Could you check a few things on this model? Use its own coordinates, in mm. Face numbers are marked on the shaded views. Round coordinates to 2 decimals unless told otherwise and drop trailing zeros. Order: outer loops, then holes, each group sorted by start corner. A loop starts at its lowest first (then second) coordinate and runs counter-clockwise, first axis right, second up. Notation, with made-up numbers: (-17, 54.25) - (-11, 54.25) arc R20 ccw to (-11, 79.25) - close; hole circle Ø1 at (21.25, -40). An arc over 180 degrees is marked (long way). Return JSON: item names as keys, results as strings. Group by question number.
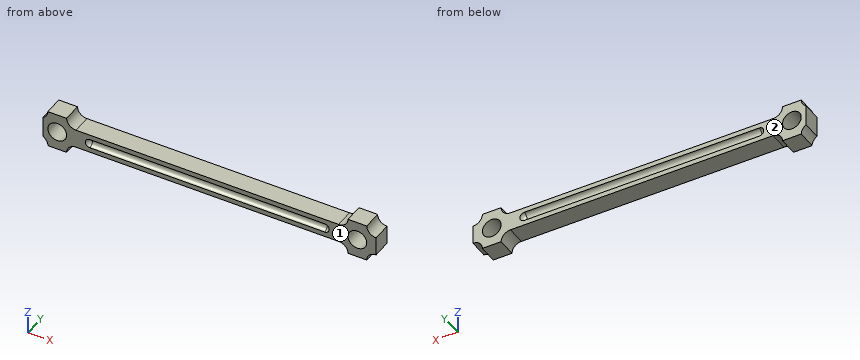
from build123d import *

# Parameters (mm, degrees)
F0_R     = 3.175
F1_DEPTH = 3.175
F3_DEPTH = 41.275
F4_R     = 1.52399


# Not quite as in the source:
# - a fillet or chamfer is up to 0.001 mm smaller than in the source, because OpenCascade refuses the exact size


with BuildPart() as f1:
    # F0 (on Front) → F1 (new body, symmetric)
    with BuildSketch(Plane.XZ):
        with BuildLine():
            Line((44.45, 3.175), (-44.45, 3.175))
            ThreePointArc((-44.45, 3.175), (-46.6950640303, 4.1049359697), (-47.625, 6.35))
            Line((-47.625, 6.35), (-53.975, 6.35))
            ThreePointArc((-53.975, 6.35), (-54.4187617277, 4.7310613044), (-55.626, 3.5646725507))
            Line((-55.626, 3.5646725507), (-55.626, -3.5646725507))
            ThreePointArc((-55.626, -3.5646725507), (-54.4187617277, -4.7310613044), (-53.975, -6.35))
            Line((-53.975, -6.35), (-47.625, -6.35))
            ThreePointArc((-47.625, -6.35), (-46.6950640303, -4.1049359697), (-44.45, -3.175))
            Line((-44.45, -3.175), (44.45, -3.175))
            ThreePointArc((44.45, -3.175), (46.6950640303, -4.1049359697), (47.625, -6.35))
            Line((47.625, -6.35), (53.975, -6.35))
            ThreePointArc((53.975, -6.35), (54.9049359697, -4.1049359697), (57.15, -3.175))
            Line((57.15, -3.175), (57.15, 3.175))
            ThreePointArc((57.15, 3.175), (54.9049359697, 4.1049359697), (53.975, 6.35))
            Line((53.975, 6.35), (47.625, 6.35))
            ThreePointArc((47.625, 6.35), (46.6950640303, 4.1049359697), (44.45, 3.175))
        make_face()
        with Locations((-50.8, 0)):
            Circle(F0_R, mode=Mode.SUBTRACT)
        with Locations((50.8, 0)):
            Circle(F0_R, mode=Mode.SUBTRACT)
    extrude(amount=F1_DEPTH, both=True)

    # F2 (on Right) → F3 (cut, symmetric)
    with BuildSketch(Plane.YZ):
        with BuildLine():
            Line((3.175, -1.524), (3.175, 1.524))
            ThreePointArc((3.175, 1.524), (1.651, 0), (3.175, -1.524))
        make_face()
        with BuildLine():
            Line((-3.175, 1.524), (-3.175, -1.524))
            ThreePointArc((-3.175, -1.524), (-1.651, 0), (-3.175, 1.524))
        make_face()
    extrude(amount=F3_DEPTH, both=True, mode=Mode.SUBTRACT)

    # F4 (radius 1.524 in the source; OpenCascade refuses exactly that, so slightly less here)
    f4_edges = [f1.edges().sort_by_distance(p)[0] for p in [
        (41.275, 1.651, 0),
        (-41.275, 1.651, 0),
        (-41.275, -1.651, 0),
        (41.275, -1.651, 0),
    ]]
    fillet(f4_edges, radius=F4_R)


solid = f1.part
1) Will this pin go through, and if not, where does the flat tip stop? pin 1 (3 mm diameter, centred on x = -19.5, y = 0.5, fed in from +Z) (3 decimals).
2) If I drill on line 1 along Z through (x, y) = (50.8, 0.5) (3 decimals); line 2 along X through (y, z) = (0.75, -1.25); line 3 along Y through (x, z) = (35, 0), over which ranges is the centre line in solid material (lowest first)? Write a range as from..to.
3) I want a section at A-A, the plane x = -50.8. List the corners of the cut face in (y, z) for me (3 decimals), plus the area to 3 significant figures.
4) I want a section at C-C, the plane x = 37. List the corners of the cut face in (y, z) for me (3 decimals), plus the area to 3 significant figures.
5) I want a section at B-B, the plane z = 4.5. List the corners of the cut face in (x, y) for me (3 decimals), plus the area to 3 significant figures.
6) We'd pull the mould along Y, two halves only. Please class the marked faces 1 and 2: +Y half, -Y half, draft (parallel to the pull), parting line (faces both ways), or undercut.
Outcome:
{
 "1": {"pin 1": "z = 3.175"},
 "2": {"line 1": "-6.35..-3.175, 3.175..6.35", "line 2": "-55.63..-53.72, -47.88..47.88, 53.72..57.15", "line 3": "-1.65..1.65"},
 "3": {"outline": "(-3.175, -6.35) - (3.175, -6.35) - (3.175, -3.175) - (-3.175, -3.175) - close; (-3.175, 3.175) - (3.175, 3.175) - (3.175, 6.35) - (-3.175, 6.35) - close", "area": "40.3 mm^2"},
 "4": {"outline": "(-3.175, -3.175) - (3.175, -3.175) - (3.175, -1.524) arc R1.524 cw to (3.175, 1.524) - (3.175, 3.175) - (-3.175, 3.175) - (-3.175, 1.524) arc R1.524 cw to (-3.175, -1.524) - close", "area": "33.0 mm^2"},
 "5": {"outline": "(-54.57, -3.175) - (-47.03, -3.175) - (-47.03, 3.175) - (-54.57, 3.175) - close; (47.03, -3.175) - (54.57, -3.175) - (54.57, 3.175) - (47.03, 3.175) - close", "area": "95.7 mm^2"},
 "6": {"face 1": "-Y half", "face 2": "+Y half"}
}
